from build123d import *

# Parameters (mm, degrees)
F0_W     = 44
F0_H     = 25.4
F1_DEPTH = 77.5
F2_R     = 3
F3_DEPTH = 25.401


with BuildPart() as f1:
    # F0 (on Front) → F1 (new body)
    with BuildSketch(Plane.XZ):
        Rectangle(F0_W, F0_H)
    extrude(amount=-F1_DEPTH)

    # F2 (on face) → F3 (cut, through all)
    with BuildSketch(Plane.XY.offset(12.7)):
        with Locations((-16, 56.75)):
            Circle(F2_R)
        with Locations((-16, 20.75)):
            Circle(F2_R)
        with Locations((16, 20.75)):
            Circle(F2_R)
        with Locations((16, 56.75)):
            Circle(F2_R)
    extrude(amount=-F3_DEPTH, mode=Mode.SUBTRACT)


solid = f1.part
Input: part model. Units: mm. Frame: model coordinates. Give positions to 0.01 mm unless a question says otherwise; leave off trailing zeros. Loops run counter-clockwise (first coordinate to the right, second up) from the corner with the lowest first, then second, coordinate; pieces in that order, holes last. Notation, with made-up numbers: M 88.25,3.5 L 133.25,3.5 A12 cw 133.25,19.5 Z; hole C -35,34.5 d9. An arc over 180 degrees is marked long. Use CSV: the item, a comma, the result in double quotes.
(1) Material intervals for L1, parallel to Y at x = 16, z = 3; L2, parallel to Y at x = 14, z = 3.25; L3, parallel to X at y = 56, z = -4.25, sorted ascending. Write a range as [from, to].
Outcome:
L1,"y = [0, 17.75], [23.75, 53.75], [59.75, 77.5]"
L2,"y = [0, 18.51], [22.99, 54.51], [58.99, 77.5]"
L3,"x = [-22, -18.9], [-13.1, 13.1], [18.9, 22]"
(2) Pin query (flat end, axial travel): P1, Ø5, axis at x = 16, y = 56.75, coming from the +Z side. Return the tip coordinate at first contact, or that it passes through.
Outcome:
P1,"passes through"
(3) Section A-A, the plane x = 16. Return loops of the section in (y, z), plus the area to 3 significant figures.
Outcome:
outline,"M 0,-12.7 L 17.75,-12.7 L 17.75,12.7 L 0,12.7 Z; M 23.75,-12.7 L 53.75,-12.7 L 53.75,12.7 L 23.75,12.7 Z; M 59.75,-12.7 L 77.5,-12.7 L 77.5,12.7 L 59.75,12.7 Z"
area,"1,660 mm²"
(4) Pull-direction query (Y, two-part tool) for faces 1 (the face through (0, 0, 0)), 2 (the face through (0, 38, 12.7)), 3 (the face through (15.609, 59.724, 0.178)), 4 (the face through (-18.997, 20.882, 0.178)); classes: pulls with the +Y half, pulls with the -Y half, needs draft (parallel to the pull), parting line crosses it, or undercut.
Outcome:
face 1,"pulls with the -Y half"
face 2,"needs draft"
face 3,"undercut"
face 4,"undercut"
(5) Section C-C, the plane z = 7.75. Return loops of the section in (x, y).
Outcome:
outline,"M -22,0 L 22,0 L 22,77.5 L -22,77.5 Z; hole C -16,20.75 d6; hole C -16,56.75 d6; hole C 16,20.75 d6; hole C 16,56.75 d6"
(6) Section B-B, the plane y = 20.75. Return loops of the section in (x, z), plus the area to 3 significant figures.
Outcome:
outline,"M -22,-12.7 L -19,-12.7 L -19,12.7 L -22,12.7 Z; M -13,-12.7 L 13,-12.7 L 13,12.7 L -13,12.7 Z; M 19,-12.7 L 22,-12.7 L 22,12.7 L 19,12.7 Z"
area,"813 mm²"
